Autodesk Inventor part; units mm, degrees
ref_plane "YZ Plane" through (0, 0, 0) normal (1, 0, 0) x (0, 1, 0)
ref_plane "XZ Plane" through (0, 0, 0) normal (0, 1, 0) x (-1, 0, 0)
ref_plane "XY Plane" through (0, 0, 0) normal (0, 0, 1) x (1, 0, 0)
sketch "Sketch1" plane through (0, 0, 0) normal (0, 0, 1) x (1, 0, 0)
  line L0 (-750, 0) -> (750, 0) construction
  line L1 (750, 0) -> (750, -2100) construction
  line L2 (750, -2100) -> (110, -2700) construction
  line L3 (108.907697, -2700) -> (-108.907697, -2700) construction
  line L4 (-110, -2700) -> (-750, -2100) construction
  line L5 (-750, -2100) -> (-750, 0) construction
  arc A0 (745.236855, 0.447083) -> (-745.236855, 0.447083) centre (0, -7964.766161) ccw construction
  arc A1 (-750.626493, -4.742884) -> (-776.293231, -222.5) centre (7180.794412, -1050) ccw construction
  arc A2 (-777.58325, -235) -> (-778.853429, -247.5) centre (7180.794412, -1050) ccw construction
  arc A3 (750.128547, -2099.028611) -> (778.853429, -247.5) centre (-7180.794412, -1050) ccw
  arc A4 (777.58325, -235) -> (776.293231, -222.5) centre (-7180.794412, -1050) ccw construction
  line L6 (-777.58325, -235) -> (777.58325, -235) construction
  arc A5 (-749.322934, -2100.70831) -> (-677.569881, -2174.801078) centre (5033.298449, 3427.518345) ccw construction
  line L7 (-750, -2100) -> (750, -2100) construction
  line L8 (-547.172872, -2035.710935) -> (-801.083389, -2306.54882) construction
  arc A6 (-677.569881, -2174.801078) -> (-110.836747, -2699.297556) centre (5033.298449, 3427.518345) ccw construction
  arc A7 (-745.236855, 0.447083) -> (-750.626493, -4.742884) centre (-744.677927, -5.526826) ccw construction
  arc A8 (750.626493, -4.742884) -> (745.236855, 0.447083) centre (744.677927, -5.526826) ccw construction
  arc A9 (-750.128547, -2099.028611) -> (-749.322934, -2100.70831) centre (-747.154451, -2098.635225) ccw construction
  arc A10 (110.836747, -2699.297556) -> (677.569881, -2174.801078) centre (-5033.298449, 3427.518345) ccw construction
  line L9 (553.81945, -2042.800618) -> (794.436811, -2299.459137) construction
  arc A11 (677.569881, -2174.801078) -> (749.322934, -2100.70831) centre (-5033.298449, 3427.518345) ccw
  arc A12 (749.322934, -2100.70831) -> (750.128547, -2099.028611) centre (747.154451, -2098.635225) ccw
  arc A13 (-110.836747, -2699.297556) -> (-108.907697, -2700) centre (-108.907697, -2697) ccw construction
  arc A14 (108.907697, -2700) -> (110.836747, -2699.297556) centre (108.907697, -2697) ccw construction
  line L10 (776.293231, -222.5) -> (-776.293231, -222.5) construction
  line L11 (778.853429, -247.5) -> (-778.853429, -247.5) construction
  arc A15 (778.853429, -247.5) -> (777.58325, -235) centre (-7180.794412, -1050) ccw
  arc A16 (776.293231, -222.5) -> (750.626493, -4.742884) centre (-7180.794412, -1050) ccw construction
  arc A17 (-776.293231, -222.5) -> (-777.58325, -235) centre (7180.794412, -1050) ccw construction
  arc A18 (-778.853429, -247.5) -> (-750.128547, -2099.028611) centre (7180.794412, -1050) ccw construction
  point P0 (0, 0)
  point P1 (0, 0)
  point P2 (0, 0)
  point P3 (0, -2700)
  point P4 (-674.128131, -2171.129877)
  point P5 (674.128131, -2171.129877)
  dimension "d43" = 1500
  dimension "d44" = 2100
  dimension "d45" = 220
  dimension "d46" = 2700
  dimension "d47" = 8000
  dimension "d48" = 8000
  dimension "d49" = 8000
  dimension "d50" = 235
  dimension "d51" = 8000
  dimension "d52" = 104
  dimension "d53" = 6
  dimension "d54" = 3
  dimension "d55" = 8000
  dimension "d56" = 104
  dimension "d57" = 3
  dimension "d67" = 12.5
  dimension "d68" = 12.5
contour flange "Contour Flange1" sketch "Sketch1" thickness 3 bend radius 3 width 1000 along (0, 0, 1) mid plane no both sides no wall seen from (713.565816, -2137.870332, 0) lies toward (0.718358, -0.6956736, 0) curves A11 A12 A3 A15
bend "Bend1"
corner "Corner1"
equation "\"d43\" = Бак_ширина_общая"
equation "\"d44\" = Бак_высота_до_конуса"
equation "\"d45\" = Бак_брюхо_ширина_полки"
equation "\"d47\" = Бак_радиус_стенок_общий"
equation "\"d48\" = Бак_радиус_стенок_общий"
equation "\"d49\" = Бак_радиус_стенок_общий"
equation "\"d50\" = Бак_спина_длина_фланцев"
equation "\"d51\" = Бак_радиус_стенок_общий"
equation "\"d53\" = d65 + d66"
equation "\"d54\" = Thickness"
equation "\"d55\" = Бак_радиус_стенок_общий"
equation "\"d67\" = Бак_нахлест_фланца"
equation "\"d68\" = Бак_нахлест_фланца"
equation "\"d8\" = Thickness"
equation "\"d9\" = BendReliefWidth"
equation "\"d10\" = BendReliefDepth"
equation "\"d11\" = MinimumRemnant"
equation "\"d12\" = TransitionRadius"
equation "\"d14\" = BendRadius"
equation "\"d16\" = CornerReliefSize"
equation "\"d17\" = GapSize"
equation "\"d18\" = JacobiRadiusSize"
equation "\"BendRadius\" = Thickness"
equation "\"BendReliefWidth\" = Thickness"
equation "\"BendReliefDepth\" = 0.5 * Thickness"
equation "\"CornerReliefSize\" = 4 * Thickness"
equation "\"MinimumRemnant\" = 2 * Thickness"
equation "\"TransitionRadius\" = BendRadius"
equation "\"JacobiRadiusSize\" = BendRadius"
equation "\"GapSize\" = Thickness"
equation "\"d66\" = d65"
properties part number "МОО 020 лист борт 1"
Check sheet for the modelled part. Datum: model origin and axes. Units: mm. Round coordinates to 2 decimals unless told otherwise and drop trailing zeros. Order: outer loops, then holes, each group sorted by start corner. A loop starts at its lowest first (then second) coordinate and runs counter-clockwise, first axis right, second up. Notation, with made-up numbers: M 75,64.25 L 113,64.25 A20 cw 113,101.25 Z; hole C -11,42 d10. An arc over 180 degrees is marked long. One line per item, written item: value. Start each with the question number.
1. Section check B-B on y = -792.5. Enter the section's corners in (x, z).
2. Section check C-C on x = 704.5. Enter the section's corners in (y, z), and give its area (3 significant figures).
3. Section check A-A on z = 758. Enter the section's corners in (x, y).
4. Gauge pin test, flat ends, axial feed: P1, Ø12, axis at x = 734, z = 406.5, coming from the +Y side; P2, Ø1.5, axis at y = -1715, z = 357.5, coming from the -X side; P3, Ø6, axis at x = 708, z = 267.5, coming from the +Y side. Record the tip position at first contact, or that the pin passes through.
5. Scan lines: line 1 along X through (y, z) = (-1088, 213); line 2 along X through (y, z) = (-1862, 635); line 3 along Y through (x, z) = (692, 537). Record each from-to range of solid material in increasing order.
Results found:
1. outline: M 815.06,0 L 818.06,0 L 818.06,1000 L 815.06,1000 Z
2. outline: M -2151.52,0 L -2147.22,0 L -2147.22,1000 L -2151.52,1000 Z
2. area: 4,300 mm^2
3. outline: M 677.57,-2174.8 L 679.71,-2176.9 A8003.01 ccw 751.49,-2102.78 A6 ccw 753.1,-2099.42 A8003 ccw 781.84,-247.2 A8003.84 ccw 780.57,-234.69 L 777.58,-235 A8000.84 cw 778.85,-247.5 A8000 cw 750.13,-2099.03 A3 cw 749.32,-2100.71 A8000.01 cw Z
4. P1: y = -2110.44
4. P2: x = 791.46
4. P3: y = -2140.52
5. line 1: 819.12 to 822.12
5. line 2: 777.89 to 780.91
5. line 3: -2164.35 to -2160.05
